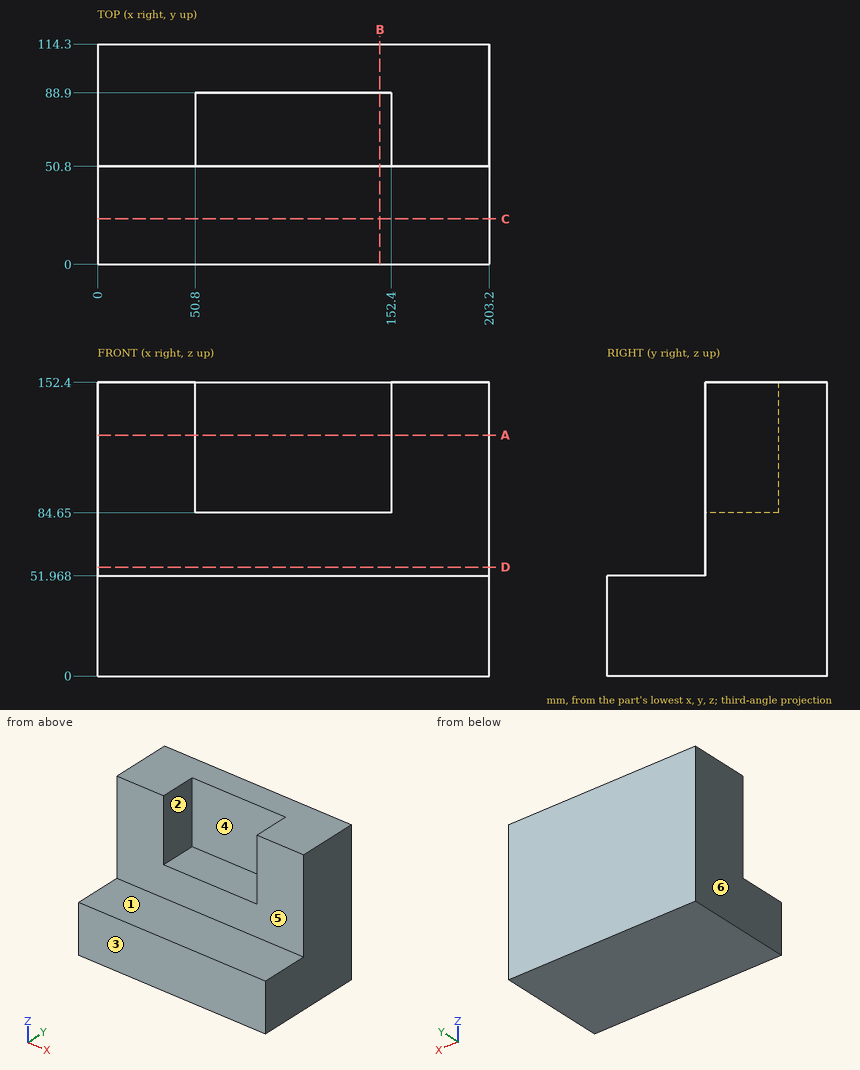
Input: dimensioned drawing with shaded views. Units: mm. Origin: part minimum x, y, z. A direction names the side the tool comes from. Round coordinates to 2 decimals unless told otherwise and drop trailing zeros. Order: outer loops, then holes, each group sorted by start corner. A loop starts at its lowest first (then second) coordinate and runs counter-clockwise, first axis right, second up. Notation, with made-up numbers: (86.5, 13) - (136.5, 13) arc R22 cw to (136.5, 25) - close; hole circle Ø2 at (-23, 81). An arc over 180 degrees is marked (long way). Answer as a JSON object with one key per item and string values. Group by question number.
(1) Cut plane C-C (y = 23.5). Return loops of the section in (x, z).
(2) Cut plane A-A (z = 125). Return loops of the section in (x, y).
(3) Reachability of the marked faces 1, 2 and 3 from +Z, -Z, +X, -X, +Y, -Y: full face, straight path, thin tool, end or side. Return the list, or none.
(4) Pin query (flat end, axial travel): P1, Ø8, axis at x = 85.5, z = 94.5, coming from the -Y side; P2, Ø3, axis at x = 160.5, y = 17.5, coming from the +Z side; P3, Ø12, axis at x = 117.5, z = 71, coming from the -Y side. Return the tip coordinate at first contact, or that it passes through.
(5) Cut plane B-B (x = 146.5). Return loops of the section in (y, z).
(6) Draft query along X for the marked faces 4, 5 and 6. Return one class per face: released by +X, released by -X, zero draft, split by the parting line, or undercut.
(7) Cut plane D-D (z = 56.5). Return loops of the section in (x, y).
(8) Material intervals for probe 1 along Y at (x, z) = (140.5, 107.5); probe 2 along Z at (x, y) = (182, 30.5); probe 3 along Y at (x, z) = (15.5, 136.5), sorted ascending. Write a range as from..to.
Here are the results:
{
 "1": {"outline": "(0, 0) - (203.2, 0) - (203.2, 51.97) - (0, 51.97) - close"},
 "2": {"outline": "(0, 50.8) - (50.8, 50.8) - (50.8, 88.9) - (152.4, 88.9) - (152.4, 50.8) - (203.2, 50.8) - (203.2, 114.3) - (0, 114.3) - close"},
 "3": {"face 1": "+Z, +X, -X, -Y", "face 2": "+Z, -Y", "face 3": "+Z, -Z, +X, -X, -Y"},
 "4": {"P1": "stops at y = 88.9", "P2": "stops at z = 51.97", "P3": "stops at y = 50.8"},
 "5": {"outline": "(0, 0) - (114.3, 0) - (114.3, 152.4) - (88.9, 152.4) - (88.9, 84.65) - (50.8, 84.65) - (50.8, 51.97) - (0, 51.97) - close"},
 "6": {"face 4": "undercut", "face 5": "zero draft", "face 6": "released by -X"},
 "7": {"outline": "(0, 50.8) - (203.2, 50.8) - (203.2, 114.3) - (0, 114.3) - close"},
 "8": {"probe 1": "y = 88.9..114.3", "probe 2": "z = 0..51.97", "probe 3": "y = 50.8..114.3"}
}
